Source: three-view drawing plus pictorial views. Frame: mm from the lowest corner of the part. A direction names the side the tool comes from. Give positions to 0.01 mm unless a question says otherwise; leave off trailing zeros. Order: outer loops, then holes, each group sorted by start corner. A loop starts at its lowest first (then second) coordinate and runs counter-clockwise, first axis right, second up. Notation, with made-up numbers: (42, 82.25) - (79, 82.25) arc R22 ccw to (79, 102.25) - close; hole circle Ø3 at (76.5, 60.5). An arc over 180 degrees is marked (long way). Use CSV: the item, a comma, the result in double quotes.
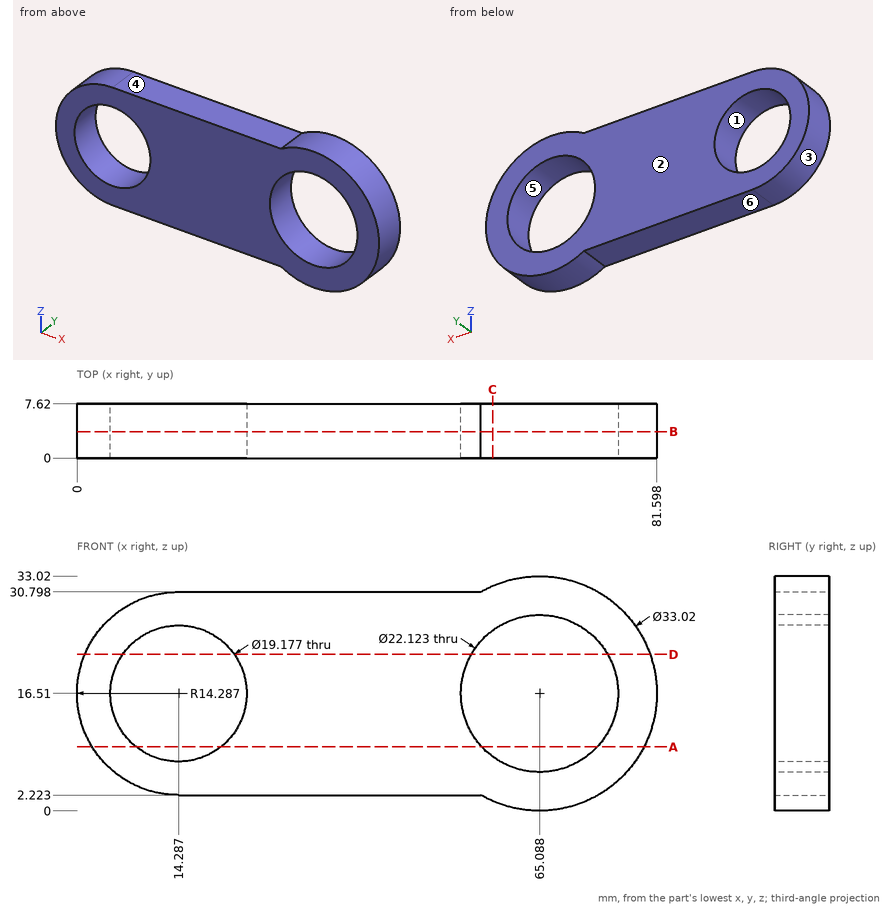
Item 1: Mould query, pull axis X, two halves, no side actions, for the marked faces 1, 2 and 3. Classes: released by +X, released by -X, zero draft, split by the parting line, or undercut.
Filled in:
face 1,"undercut"
face 2,"zero draft"
face 3,"released by -X"
Item 2: First-contact query: pin 1 (1 mm diameter, centred on y = 3, z = 7.5, fed in from +X) (1 decimal); pin 2 (12 mm diameter, centred on x = 67, z = 16, fed in from +Y); pin 3 (2 mm diameter, centred on y = 6.5, z = 8.5, fed in from -X); pin 4 (1 mm diameter, centred on y = 2.5, z = 15, fed in from -X). Flat tips, straight axial feed; report the tip coordinate or a pass-through.
Filled in:
pin 1,"stops at x = 79.2"
pin 2,"passes through"
pin 3,"stops at x = 1.84"
pin 4,"stops at x = 0.04"
Item 3: Section A-A on z = 9. Return the cut outline in (x, y) (1 decimal).
Filled in:
outline,"(2.1, 0) - (8.3, 0) - (8.3, 7.6) - (2.1, 7.6) - close; (20.2, 0) - (57, 0) - (57, 7.6) - (20.2, 7.6) - close; (73.2, 0) - (79.8, 0) - (79.8, 7.6) - (73.2, 7.6) - close"
Item 4: Section D-D on z = 22. Return the cut outline in (x, y) (1 decimal), then the cut area to 3 significant figures.
Filled in:
outline,"(1.1, 0) - (6.4, 0) - (6.4, 7.6) - (1.1, 7.6) - close; (22.1, 0) - (55.5, 0) - (55.5, 7.6) - (22.1, 7.6) - close; (74.7, 0) - (80.7, 0) - (80.7, 7.6) - (74.7, 7.6) - close"
area,"340 mm2"
Item 5: Set-up query: the marked faces 4, 5 and 6. Return all of +Z, -Z, +X, -X, +Y, -Y with unobstructed straight access to the full face (end or side cutting, diameter ignored); none if empty.
Filled in:
face 4,"+Z, -X, +Y, -Y"
face 5,"+Y, -Y"
face 6,"-Z, -X, +Y, -Y"
Item 6: Section C-C on x = 58.5. Return the cut outline in (y, z).
Filled in:
outline,"(0, 1.37) - (7.62, 1.37) - (7.62, 7.62) - (0, 7.62) - close; (0, 25.4) - (7.62, 25.4) - (7.62, 31.65) - (0, 31.65) - close"
Item 7: Section B-B on y = 3.75. Return the cut outline in (x, z) (1 decimal), then the cut area to 3 significant figures.
Filled in:
outline,"(14.3, 2.2) - (56.8, 2.2) arc R16.5 ccw (long way) to (56.8, 30.8) - (14.3, 30.8) arc R14.3 ccw to start; hole circle Ø19.2 at (14.3, 16.5); hole circle Ø22.1 at (65.1, 16.5)"
area,"1,550 mm2"
Item 8: Material intervals for line 1 (X direction, y = 6.25, z = 17); line 2 (X direction, y = 2, z = 15.5) (1 decimal); line 3 (Z direction, x = 36.5, y = 6), sorted ascending. Write a range as from..to.
Filled in:
line 1,"x = 0.01..4.71, 23.86..54.04, 76.14..81.59"
line 2,"x = 0..4.8, 23.8..54.1, 76.1..81.6"
line 3,"z = 2.22..30.8"
